Work out the finished part from the listing and answer in its coordinate system (mm). Face numbers are marked on the shaded views. A direction names the side the tool comes from. Round coordinates to 2 decimals unless told otherwise and drop trailing zeros. Loops run counter-clockwise (first coordinate to the right, second up) from the corner with the lowest first, then second, coordinate; pieces in that order, holes last. Notation, with made-up numbers: (-18.5, 26.5) - (29.5, 26.5) arc R27 cw to (29.5, 44.5) - close; hole circle Ø11 at (75, -40). An arc over 180 degrees is marked (long way). Answer as CSV lines item,"result". Start each with the question number.
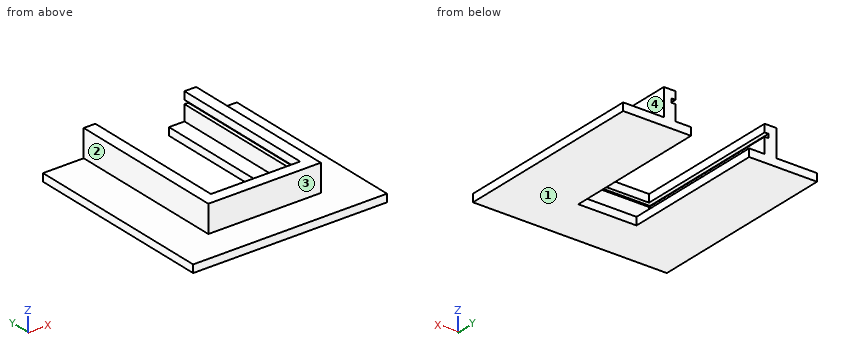
Autodesk Inventor part; units mm, degrees
ref_plane "YZ Plane" through (0, 0, 0) normal (1, 0, 0) x (0, 1, 0)
ref_plane "XZ Plane" through (0, 0, 0) normal (0, 1, 0) x (-1, 0, 0)
ref_plane "XY Plane" through (0, 0, 0) normal (0, 0, 1) x (1, 0, 0)
sketch "Skizze4" plane through (0, 0, 0) normal (0, 0, 1) x (1, 0, 0)
  line L0 (0, 0) -> (50, 0)
  line L1 (50, 0) -> (50, 50)
  line L2 (50, 50) -> (0, 50)
  line L3 (0, 50) -> (0, 0)
  dimension "d5" = 50
  dimension "d6" = 50
extrude "Extrusion1" add sketch "Skizze4" along normal blind 2
sketch "Skizze5" plane through (0, 0, 2) normal (0, 0, 1) x (1, 0, 0)
  line L0 (50, 50) -> (0, 50)
  line L1 (17.5, 50) -> (32.5, 50)
  line L2 (32.5, 50) -> (32.5, 12.5)
  line L3 (32.5, 12.5) -> (17.5, 12.5)
  line L4 (17.5, 12.5) -> (17.5, 50)
  point P0 (0, 0)
  dimension "d10" = 15
  dimension "d11" = 37.5
extrude "Extrusion2" cut sketch "Skizze5" against normal blind 2
sketch "Skizze6" plane through (0, 0, 2) normal (0, 0, 1) x (1, 0, 0)
  line L0 (17.5, 50) -> (0, 50)
  line L1 (12.5, 50) -> (10.5, 50)
  line L2 (10.5, 50) -> (10.5, 10.5)
  line L3 (10.5, 10.5) -> (12.5, 10.5)
  line L4 (12.5, 12.5) -> (12.5, 50)
  line L5 (10.5, 10.5) -> (39.5, 10.5)
  line L6 (39.5, 10.5) -> (39.5, 12.5)
  line L7 (37.5, 12.5) -> (12.5, 12.5)
  line L8 (10.5, 12.5) -> (10.5, 10.5)
  line L9 (50, 50) -> (32.5, 50)
  line L10 (39.5, 10.5) -> (37.5, 10.5)
  line L11 (37.5, 12.5) -> (37.5, 50)
  line L12 (37.5, 50) -> (39.5, 50)
  line L13 (39.5, 50) -> (39.5, 10.5)
  point P0 (0, 0)
  dimension "d14" = 2
  dimension "d15" = 39.5
  dimension "d16" = 29
  dimension "d17" = 2
  dimension "d18" = 2
extrude "Extrusion3" add sketch "Skizze6" along normal blind 9
sketch "Skizze7" plane through (37.5, 12.5, 2) normal (-1, 0, 0) x (0, 0, 1)
  line L0 (0, -12.5) -> (0, 37.5)
  line L1 (9, 37.5) -> (0, 37.5)
  line L2 (0, 37.5) -> (0, 0)
  line L3 (0, 0) -> (9, 0)
  line L4 (9, 0) -> (9, 37.5)
  point P0 (-2, -12.5)
  dimension "d21" = 37.5
extrude "Extrusion4" add sketch "Skizze7" along normal blind 2
sketch "Skizze9" plane through (35.5, 12.5, 2) normal (-1, 0, 0) x (0, 0, 1)
  line L0 (9, 0) -> (0, 0)
  line L1 (7, 37.5) -> (6, 37.5)
  line L2 (6, 37.5) -> (6, 0)
  line L3 (6, 0) -> (7, 0)
  line L4 (7, 0) -> (7, 37.5)
  point P0 (-2, -12.5)
  dimension "d24" = 1
extrude "Extrusion5" cut sketch "Skizze9" against normal blind 1
sketch "Skizze10" plane through (17.5, 12.5, 0) normal (0, 1, 0) x (1, 0, 0)
  line L0 (18, -2) -> (-5, -2)
  line L1 (-5, -2) -> (-5, -11)
  line L2 (-5, -11) -> (18, -11)
  line L3 (18, -11) -> (18, -2)
  point P0 (-17.5, 0)
extrude "Extrusion6" add sketch "Skizze10" along normal blind 2
sketch "Skizze11" plane through (17.5, 14.5, 0) normal (0, 1, 0) x (1, 0, 0)
  line L0 (-5, -11) -> (-5, -2)
  line L1 (19, -9) -> (-5, -9)
  line L2 (-5, -9) -> (-5, -8)
  line L3 (-5, -8) -> (19, -8)
  line L4 (19, -8) -> (19, -9)
  point P0 (-17.5, 0)
extrude "Extrusion7" cut sketch "Skizze11" against normal blind 1
sketch "Skizze12" plane through (36.5, 12.5, 9) normal (0, 1, 0) x (1, 0, 0)
  line L0 (-1, 1) -> (0, 1)
  line L1 (0, 1) -> (0, 0)
  line L2 (0, 0) -> (-1, 0)
  line L3 (-1, 0) -> (-1, 1)
  point P0 (-36.5, 9)
extrude "Extrusion8" add sketch "Skizze12" along normal blind 1
sketch "Skizze13" plane through (12.5, 50, 11) normal (1, 0, 0) x (0, 0, -1)
  line L0 (9, -35.5) -> (9, -37.5)
  line L1 (0, 0) -> (9, 0)
  line L2 (9, 0) -> (9, -36.5)
  line L3 (9, -36.5) -> (0, -36.5)
  line L4 (0, -36.5) -> (0, 0)
  point P0 (11, -50)
extrude "Extrusion9" add sketch "Skizze13" along normal blind 2
sketch "Skizze14" plane through (14.5, 50, 11) normal (1, 0, 0) x (0, 0, -1)
  line L0 (9, 0) -> (0, 0)
  line L1 (2, 0) -> (3, 0)
  line L2 (3, 0) -> (3, -37.5)
  line L3 (3, -37.5) -> (2, -37.5)
  line L4 (2, -37.5) -> (2, 0)
  point P0 (11, -50)
  dimension "d35" = 1
  dimension "d36" = 37.5
extrude "Extrusion10" cut sketch "Skizze14" against normal blind 1
sketch "Skizze15" plane through (10.5, 10.5, 2) normal (0, -1, 0) x (1, 0, 0)
  line L0 (0, 9) -> (29, 9)
  line L1 (29, 9) -> (29, 0)
  line L2 (29, 0) -> (0, 0)
  line L3 (0, 0) -> (0, 9)
  point P0 (-10.5, -2)
extrude "Extrusion11" add sketch "Skizze15" along normal blind 2
sketch "Skizze16" plane through (17.5, 14.5, 0) normal (0, 1, 0) x (1, 0, 0)
  line L0 (-3, -2) -> (18, -2)
  line L1 (18, -2) -> (18, -8)
  line L2 (18, -8) -> (-3, -8)
  line L3 (-3, -8) -> (-3, -2)
  point P0 (-17.5, 0)
extrude "Extrusion12" cut sketch "Skizze16" against normal blind 4
sketch "Skizze17" plane through (17.5, 13.5, 0) normal (0, 1, 0) x (1, 0, 0)
  line L0 (-3, -8) -> (19, -8)
  line L1 (19, -8) -> (19, -9)
  line L2 (19, -9) -> (-3, -9)
  line L3 (-3, -9) -> (-3, -8)
  point P0 (-17.5, 0)
extrude "Extrusion13" cut sketch "Skizze17" against normal blind 2
sketch "Skizze18" plane through (14.5, 12.5, 9) normal (0, 1, 0) x (1, 0, 0)
  line L0 (0, 1) -> (-1, 1)
  line L1 (-1, 1) -> (-1, 0)
  line L2 (-1, 0) -> (0, 0)
  line L3 (0, 0) -> (0, 1)
  point P0 (-14.5, 9)
extrude "Extrusion14" cut sketch "Skizze18" against normal blind 2
sketch "Skizze19" plane through (17.5, 11.5, 0) normal (0, 1, 0) x (1, 0, 0)
  line L0 (-3, -8) -> (19, -8)
  line L1 (19, -8) -> (19, -9)
  line L2 (19, -9) -> (-3, -9)
  line L3 (-3, -9) -> (-3, -8)
  point P0 (-17.5, 0)
extrude "Extrusion15" cut sketch "Skizze19" against normal blind 1
sketch "Skizze20" plane through (36.5, 12.5, 2) normal (-1, 0, 0) x (0, 0, 1)
  line L0 (6, 37.5) -> (7, 37.5)
  line L1 (7, 37.5) -> (7, -2)
  line L2 (7, -2) -> (6, -2)
  line L3 (6, -2) -> (6, 37.5)
  point P0 (-2, -12.5)
  dimension "d49" = 39.5
extrude "Extrusion16" cut sketch "Skizze20" against normal blind 1
sketch "Skizze21" plane through (35.5, 12.5, 2) normal (-1, 0, 0) x (0, 0, 1)
  line L0 (6, 37.5) -> (6, -2)
  line L1 (0, 37.5) -> (6, 37.5)
  line L2 (6, 37.5) -> (6, -1)
  line L3 (6, -1) -> (0, -1)
  line L4 (0, -1) -> (0, 37.5)
  point P0 (-2, -12.5)
  dimension "d52" = 38.5
extrude "Extrusion17" cut sketch "Skizze21" against normal blind 1
sketch "Skizze22" plane through (35.5, 12.5, 2) normal (-1, 0, 0) x (0, 0, 1)
  line L0 (7, 37.5) -> (9, 37.5)
  line L1 (9, 37.5) -> (9, -1)
  line L2 (9, -1) -> (7, -1)
  line L3 (7, -1) -> (7, 37.5)
  point P0 (-2, -12.5)
  dimension "d55" = 38.5
extrude "Extrusion18" cut sketch "Skizze22" against normal blind 1
sketch "Skizze23" plane through (13.5, 50, 11) normal (1, 0, 0) x (0, 0, -1)
  line L0 (2, 0) -> (3, 0)
  line L1 (3, 0) -> (3, -39.5)
  line L2 (3, -39.5) -> (2, -39.5)
  line L3 (2, -39.5) -> (2, 0)
  point P0 (11, -50)
  dimension "d58" = 39.5
extrude "Extrusion19" cut sketch "Skizze23" against normal blind 1
sketch "Skizze24" plane through (14.5, 50, 11) normal (1, 0, 0) x (0, 0, -1)
  line L0 (9, -41.5) -> (9, 0)
  line L1 (3, 0) -> (9, 0)
  line L2 (9, 0) -> (9, -38.5)
  line L3 (9, -38.5) -> (3, -38.5)
  line L4 (3, -38.5) -> (3, 0)
  point P0 (11, -50)
  dimension "d62" = 38.5
extrude "Extrusion20" cut sketch "Skizze24" against normal blind 1
sketch "Skizze25" plane through (14.5, 50, 11) normal (1, 0, 0) x (0, 0, -1)
  line L0 (2, -39.5) -> (2, 0)
  line L1 (0, 0) -> (2, 0)
  line L2 (2, 0) -> (2, -38.5)
  line L3 (2, -38.5) -> (0, -38.5)
  line L4 (0, -38.5) -> (0, 0)
  point P0 (11, -50)
  dimension "d65" = 38.5
extrude "Extrusion21" cut sketch "Skizze25" against normal blind 1
sketch "Skizze26" plane through (17.5, 14.5, 0) normal (0, 1, 0) x (1, 0, 0)
  line L0 (-3, -11) -> (18, -11)
  line L1 (18, -11) -> (18, -9)
  line L2 (18, -9) -> (-3, -9)
  line L3 (-3, -9) -> (-3, -11)
  point P0 (-17.5, 0)
extrude "Extrusion22" cut sketch "Skizze26" against normal blind 3
sketch "Skizze27" plane through (14.5, 11.5, 8) normal (0, 1, 0) x (1, 0, 0)
  line L0 (0, 0) -> (-1, 0)
  line L1 (-1, 0) -> (-1, 6)
  line L2 (-1, 6) -> (0, 6)
  line L3 (0, 6) -> (0, 0)
  point P0 (-14.5, 8)
extrude "Extrusion23" cut sketch "Skizze27" against normal blind 1
sketch "Skizze28" plane through (35.5, 11.5, 8) normal (0, 1, 0) x (1, 0, 0)
  line L0 (1, 6) -> (0, 6)
  line L1 (0, 6) -> (0, 0)
  line L2 (0, 0) -> (1, 0)
  line L3 (1, 0) -> (1, 6)
  point P0 (-35.5, 8)
extrude "Extrusion24" cut sketch "Skizze28" against normal blind 1
sketch "Skizze29" plane through (17.5, 10.5, 0) normal (0, 1, 0) x (1, 0, 0)
  point P0 (-17.5, 0)
sketch "Skizze30" plane through (17.5, 10.5, 0) normal (0, 1, 0) x (1, 0, 0)
  line L0 (19, -8) -> (-4, -8)
  line L1 (-4, -8) -> (-4, -2)
  line L2 (-4, -2) -> (19, -2)
  line L3 (19, -2) -> (19, -8)
  point P0 (-17.5, 0)
extrude "Extrusion25" add sketch "Skizze30" along normal blind 1
sketch "Skizze31" plane through (0, 0, 0) normal (0, 0, -1) x (-1, 0, 0)
  line L0 (0, 50) -> (-17.5, 50)
  line L1 (-17.5, 50) -> (-17.5, 12.5)
  line L2 (0, 12.5) -> (0, 50)
  line L3 (-17.5, 12.5) -> (-32.5, 12.5)
  line L4 (-50, 12.5) -> (-50, 0)
  line L5 (-50, 0) -> (0, 0)
  line L6 (0, 0) -> (0, 12.5)
  line L7 (-32.5, 12.5) -> (-32.5, 50)
  line L8 (-32.5, 50) -> (-50, 50)
  line L9 (-50, 50) -> (-50, 12.5)
extrude "Extrusion26" cut sketch "Skizze31" against normal blind 1
sketch "Skizze32" plane through (0, 0, 2) normal (0, 0, 1) x (1, 0, 0)
  line L0 (50, 50) -> (39.5, 50)
  line L1 (39.5, 50) -> (39.5, 8.5)
  line L2 (39.5, 0) -> (50, 0)
  line L3 (50, 0) -> (50, 50)
  line L4 (50, 0) -> (0, 0)
  line L5 (0, 0) -> (0, 8.5)
  line L6 (10.5, 8.5) -> (39.5, 8.5)
  line L7 (50, 8.5) -> (50, 0)
  line L8 (10.5, 8.5) -> (10.5, 50)
  line L9 (10.5, 50) -> (0, 50)
  line L10 (0, 50) -> (0, 8.5)
extrude "Extrusion27" add sketch "Skizze32" along normal blind 2
sketch "Skizze33" plane through (0, 0, 2) normal (0, 0, 1) x (1, 0, 0)
  line L0 (17.5, 50) -> (17.5, 12.5)
  line L1 (17.5, 12.5) -> (32.5, 12.5)
  line L2 (32.5, 12.5) -> (32.5, 50)
  line L3 (32.5, 50) -> (32.5, 12.5)
  line L4 (32.5, 50) -> (36.5, 50)
  line L5 (36.5, 50) -> (36.5, 11.5)
  line L6 (36.5, 11.5) -> (36.5, 50)
  line L7 (36.5, 11.5) -> (13.5, 11.5)
  line L8 (13.5, 11.5) -> (13.5, 50)
  line L9 (17.5, 50) -> (13.5, 50)
  line L10 (13.5, 50) -> (17.5, 50)
  point P0 (0, 0)
extrude "Extrusion28" add sketch "Skizze33" along normal blind 2 and the other way blind 1
sketch "Skizze34" plane through (0, 0, 1) normal (0, 0, -1) x (-1, 0, 0)
  line L0 (-32.5, 50) -> (-50, 50)
  line L1 (-50, 50) -> (-50, 0)
  line L2 (-50, 0) -> (0, 0)
  line L3 (0, 0) -> (0, 50)
  line L4 (0, 50) -> (-17.5, 50)
  line L5 (-17.5, 50) -> (-17.5, 12.5)
  line L6 (-17.5, 12.5) -> (-32.5, 12.5)
  line L7 (-32.5, 12.5) -> (-32.5, 50)
extrude "Extrusion29" cut sketch "Skizze34" against normal blind 1
properties part number "Halterung Merkruphy"
Item 1: Section B-B, the plane z = 4.75 is taken. Give the vertices of the cut face in (x, y).
Item 2: Find the intervals of material crossed by L1, parallel to X at y = 27, z = 3.75; L2, parallel to X at y = 29.5, z = 5.5; L3, parallel to Y at x = 20, z = 9.25, in increasing order.
Item 3: Which of the six approach directions +Z, -Z, +X, -X, +Y, -Y give full straight-line access (tool end or side, diameter ignored) to the marked faces 1, 2, 3 and 4?
Item 4: Section D-D, the plane y = 7 is taken. Give the vertices of the cut face in (x, z).
Item 5: Flat-ended cylindrical pins translate along their axes: pin 1 Ø1.2 at (x, z) = (29, 6.5) entering from +Y; pin 2 Ø1 at (y, z) = (40.5, 8) entering from -X; pin 3 Ø20 at (x, y) = (25.5, 35.5) entering from +Z. Find the tip coordinate at first contact, or state that the pin passes through.
Item 6: Section A-A, the plane y = 43 is taken. Give the vertices of the cut face in (x, z).
Item 7: Section C-C, the plane x = 23 is taken. Give the vertices of the cut face in (y, z), and give its area (3 significant figures).
Answer:
1,outline,"(10.5, 8.5) - (39.5, 8.5) - (39.5, 50) - (36.5, 50) - (36.5, 11.5) - (13.5, 11.5) - (13.5, 50) - (10.5, 50) - close"
2,L1,"x = 0 to 17.5, 32.5 to 50"
2,L2,"x = 10.5 to 13.5, 36.5 to 39.5"
2,L3,"y = 8.5 to 11.5"
3,face 1,"-Z, +X, -X, +Y, -Y"
3,face 2,"+Z, -X, +Y, -Y"
3,face 3,"+Z, +X, -X, -Y"
3,face 4,"+Z, +X, +Y, -Y"
4,outline,"(0, 2) - (50, 2) - (50, 4) - (0, 4) - close"
5,pin 1,"stops at y = 11.5"
5,pin 2,"stops at x = 10.5"
5,pin 3,"stops at z = 4"
6,outline,"(0, 2) - (17.5, 2) - (17.5, 4) - (13.5, 4) - (13.5, 8) - (12.5, 8) - (12.5, 9) - (13.5, 9) - (13.5, 11) - (10.5, 11) - (10.5, 4) - (0, 4) - close; (32.5, 2) - (50, 2) - (50, 4) - (39.5, 4) - (39.5, 11) - (36.5, 11) - (36.5, 9) - (37.5, 9) - (37.5, 8) - (36.5, 8) - (36.5, 4) - (32.5, 4) - close"
7,outline,"(0, 2) - (12.5, 2) - (12.5, 4) - (11.5, 4) - (11.5, 8) - (10.5, 8) - (10.5, 9) - (11.5, 9) - (11.5, 11) - (8.5, 11) - (8.5, 4) - (0, 4) - close"
7,area,"45.0 mm²"
